Geometry check sheet. Reference: the model listing, model coordinates, mm. Coordinates: 2 decimals unless noted, no trailing zeros. Loops run counter-clockwise (first coordinate to the right, second up) from the corner with the lowest first, then second, coordinate; pieces in that order, holes last. Notation, with made-up numbers: (-26.75, 35) - (-1.75, 35) arc R9 ccw to (-1.75, 51) - close; hole circle Ø9 at (16, 44.5). An arc over 180 degrees is marked (long way). Write each question's results on one line, items separated by ' | '. Start each with the question number.
(1) Go/stop test with flat-tipped pins: pin 1 Ø1 at (x, z) = (2, -142) entering from +Y; pin 2 Ø6 at (x, z) = (7.5, -305.5) entering from +Y; pin 3 Ø2 at (y, z) = (5.5, -268) entering from -X. Record where each tip stops, or that it passes through.
(2) Material ranges on probe 1 along Y at (x, z) = (0, -303.5); probe 2 along X at (y, z) = (1, -441), recorded low to high.
(3) Sectioned sample at A-A (x = 0). Enter the section's corners in (y, z), plus the area to 3 significant figures.
(4) Sectioned sample at B-B (y = 0). Enter the section's corners in (x, z).
(5) Sectioned sample at C-C (z = -447.5). Enter the section's corners in (x, y), plus the area to 3 significant figures.
from build123d import *

# Parameters (mm, degrees)
F0_R     = 9.7
F0_R_2   = 8.7
F1_DEPTH = 500
F3_DEPTH = 10
F4_DEPTH = 12.5


with BuildPart() as f1:
    # F0 (on Top) → F1 (new body)
    with BuildSketch(Plane.XY):
        Circle(F0_R)
        Circle(F0_R_2, mode=Mode.SUBTRACT)
    extrude(amount=-F1_DEPTH)

    # F0 (on Top) → F3 (join)
    with BuildSketch(Plane.XY):
        Circle(F0_R)
        Circle(F0_R_2, mode=Mode.SUBTRACT)
    extrude(amount=F3_DEPTH)

    # F2 (on Front) → F4 (cut, symmetric)
    with BuildSketch(Plane.XZ):
        with BuildLine():
            Line((-9.7, 10), (-9.7, 4.502439))
            ThreePointArc((-9.7, 4.502439), (0, 0), (9.7, 4.502439))
            Line((9.7, 4.502439), (9.7, 10))
            Line((9.7, 10), (-9.7, 10))
        make_face()
    extrude(amount=F4_DEPTH, both=True, mode=Mode.SUBTRACT)


solid = f1.part
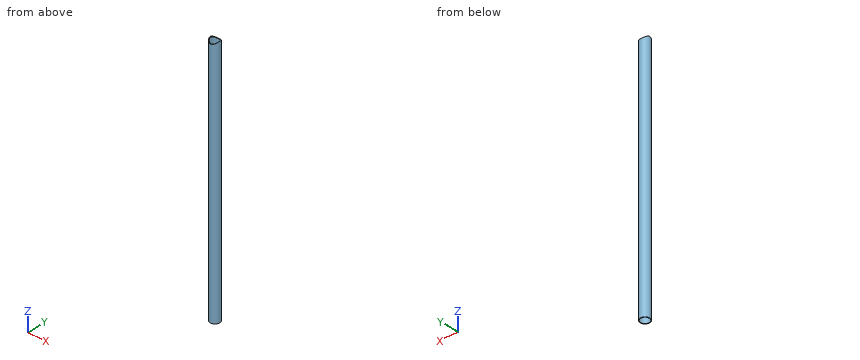
Outcome:
1) pin 1: stops at y = 9.58 | pin 2: stops at y = 8.59 | pin 3: stops at x = -8.59
2) probe 1: y = -9.7 to -8.7, 8.7 to 9.7 | probe 2: x = -9.65 to -8.64, 8.64 to 9.65
3) outline: (-9.7, -500) - (-8.7, -500) - (-8.7, 0) - (-9.7, 0) - close; (8.7, -500) - (9.7, -500) - (9.7, 0) - (8.7, 0) - close | area: 1,000 mm2
4) outline: (-9.7, -500) - (-8.7, -500) - (-8.7, 3.45) arc R12.7 cw to (-9.7, 4.5) - close; (8.7, -500) - (9.7, -500) - (9.7, 4.5) arc R12.7 cw to (8.7, 3.45) - close
5) outline: circle Ø19.4 at (0, 0); hole circle Ø17.4 at (0, 0) | area: 57.8 mm2
